Work out the finished part from the listing and answer in its coordinate system (mm). A direction names the side the tool comes from. Round coordinates to 2 decimals unless told otherwise and drop trailing zeros. Write each loop counter-clockwise with the first axis right and the second up, starting at its lowest first coordinate (ties: lowest second). Pieces come first, ordered by that corner, then holes. Notation, with made-up numbers: (-11.75, 47.5) - (17.25, 47.5) arc R16 cw to (17.25, 56.5) - close; hole circle Ø1 at (-13, 38.25). An arc over 180 degrees is marked (long way). Answer as a JSON object with one key per item and string values.
```python
from build123d import *

# Parameters (mm, degrees)
SKETCH_1_R        = 18
EXTRUDE_1_DEPTH   = 22
SKETCH_2_R        = 15.5
EXTRUDE_2_DEPTH   = 22
SKETCH_3_R        = 5
EXTRUDE_4_DEPTH   = 3
SKETCH_4_R        = 2.5
EXTRUDE_5_DEPTH   = 12
SKETCH_5_R        = 5.5
EXTRUDE_6_DEPTH   = 6
EXTRUDE_1_2_DEPTH = 5.003884266
SKETCH_7_W        = 10
SKETCH_7_H        = 4
EXTRUDE_7_DEPTH   = 4


with BuildPart() as part:
    # 草图1 → Extrude 1 (new body)
    with BuildSketch(Plane(origin=(0, 0, 0), x_dir=(1, 0, 0), z_dir=(0, 1, 0))):
        Circle(SKETCH_1_R)
    extrude(amount=EXTRUDE_1_DEPTH)

    # 草图2 → 凸台-拉伸2 (add)
    with BuildSketch(Plane(origin=(0, 22, 0), x_dir=(1, 0, 0), z_dir=(0, 1, 0))):
        Circle(SKETCH_2_R)
    extrude(amount=EXTRUDE_2_DEPTH)

    # 草图3 → 凸台-拉伸4 (add)
    with BuildSketch(Plane.XZ):
        with Locations((7.987474049, 0)):
            Circle(SKETCH_3_R)
    extrude(amount=EXTRUDE_4_DEPTH)

    # 草图4 → 凸台-拉伸5 (add)
    with BuildSketch(Plane.XZ.offset(3)):
        with Locations((7.884702341, 0)):
            Circle(SKETCH_4_R)
    extrude(amount=EXTRUDE_5_DEPTH)

    # 草图5 → 凸台-拉伸6 (add)
    with BuildSketch(Plane(origin=(0, 44, 0), x_dir=(1, 0, 0), z_dir=(0, 1, 0))):
        Circle(SKETCH_5_R)
    extrude(amount=EXTRUDE_6_DEPTH)

    # 草图6 → Extrude 1 2 (add)
    with BuildSketch(Plane(origin=(0, 44, 0), x_dir=(1, 0, 0), z_dir=(0, 1, 0))):
        Polygon((-4.778535484, 6.653759351), (-2.666405598, 8.001927364), (-2.128370145, 7.159005154), (-4.240500031, 5.810837142), align=None)
        Polygon((5.223428842, 7.129609036), (6.568517474, 5.022303512), (5.725595265, 4.484268059), (4.380506633, 6.591573583), align=None)
    extrude(amount=EXTRUDE_1_2_DEPTH)

    # 草图7 → 凸台-拉伸7 (add)
    with BuildSketch(Plane(origin=(0, 44, 0), x_dir=(1, 0, 0), z_dir=(0, 1, 0))):
        with Locations((0.014439493, -9.155250873)):
            Rectangle(SKETCH_7_W, SKETCH_7_H)
    extrude(amount=EXTRUDE_7_DEPTH)


solid = part.part
```
Item 1: Determine the mould class of faces 1 (the flat face through (5.062, 46.467, -5.523)), 2 (the flat face through (-3.737, 46.467, -7.318)), 3 (the flat face through (0, 50, 0)) for opening direction Z: pulls with the +Z half, pulls with the -Z half, needs draft (parallel to the pull), parting line crosses it, or undercut.
Results found:
{"face 1": "undercut", "face 2": "pulls with the -Z half", "face 3": "needs draft"}
Item 2: Each of these flat-tipped pins is pushed along its axis until it touches: P1, Ø1.5, axis at y = -8.5, z = 2, coming from the +X side; P2, Ø2, axis at y = 45.5, z = 9.5, coming from the -X side; P3, Ø1, axis at x = -11.5, z = 13, coming from the -Y side. Where does it stop, or does it pass through?
Results found:
{"P1": "x = 10.05", "P2": "x = -4.99", "P3": "y = 0"}
Item 3: A cutting plane is placed at A-A (y = 46.5). Write down the section's boundary in (x, z).
Results found:
{"outline": "circle Ø11 at (0, 0); (-4.99, 7.16) - (5.01, 7.16) - (5.01, 11.16) - (-4.99, 11.16) - close; (-4.78, -6.65) - (-2.67, -8) - (-2.13, -7.16) - (-4.24, -5.81) - close; (4.38, -6.59) - (5.22, -7.13) - (6.57, -5.02) - (5.73, -4.48) - close"}
Item 4: Consider line 1 along X through (y, z) = (20, -0.5); line 2 along Y through (x, z) = (-11, -9.5); line 3 along X through (y, z) = (47.5, 9). Determine where each line is inside the solid, lowest interval first.
Results found:
{"line 1": "-17.99 to 17.99", "line 2": "0 to 44", "line 3": "-4.99 to 5.01"}
Item 5: A cutting plane is placed at C-C (z = 0). Write down the section's boundary in (x, y), and give its area (3 significant figures).
Results found:
{"outline": "(-18, 0) - (2.99, 0) - (2.99, -3) - (5.38, -3) - (5.38, -15) - (10.38, -15) - (10.38, -3) - (12.99, -3) - (12.99, 0) - (18, 0) - (18, 22) - (15.5, 22) - (15.5, 44) - (5.5, 44) - (5.5, 50) - (-5.5, 50) - (-5.5, 44) - (-15.5, 44) - (-15.5, 22) - (-18, 22) - close", "area": "1,630 mm²"}
Item 6: For faces 4 (the flat face through (0, 46, 7.155)), 5 (the flat face through (5.887, 46.467, -6.091)), 6 (the flat face through (10, -3, -2)), determine the directions among +Z, -Z, +X, -X, +Y, -Y from which every point of the face is accessible in a straight line to the end or side of a thin tool.
Results found:
{"face 4": "+X, -X, +Y", "face 5": "-Z, +X, +Y", "face 6": "-Y"}
Item 7: A cutting plane is placed at B-B (x = 0). Write down the section's boundary in (y, z).
Results found:
{"outline": "(0, -18) - (22, -18) - (22, -15.5) - (44, -15.5) - (44, -5.5) - (50, -5.5) - (50, 5.5) - (44, 5.5) - (44, 7.16) - (48, 7.16) - (48, 11.16) - (44, 11.16) - (44, 15.5) - (22, 15.5) - (22, 18) - (0, 18) - close"}
Item 8: A cutting plane is placed at D-D (y = 34). Write down the section's boundary in (x, z).
Results found:
{"outline": "circle Ø31 at (0, 0)"}
